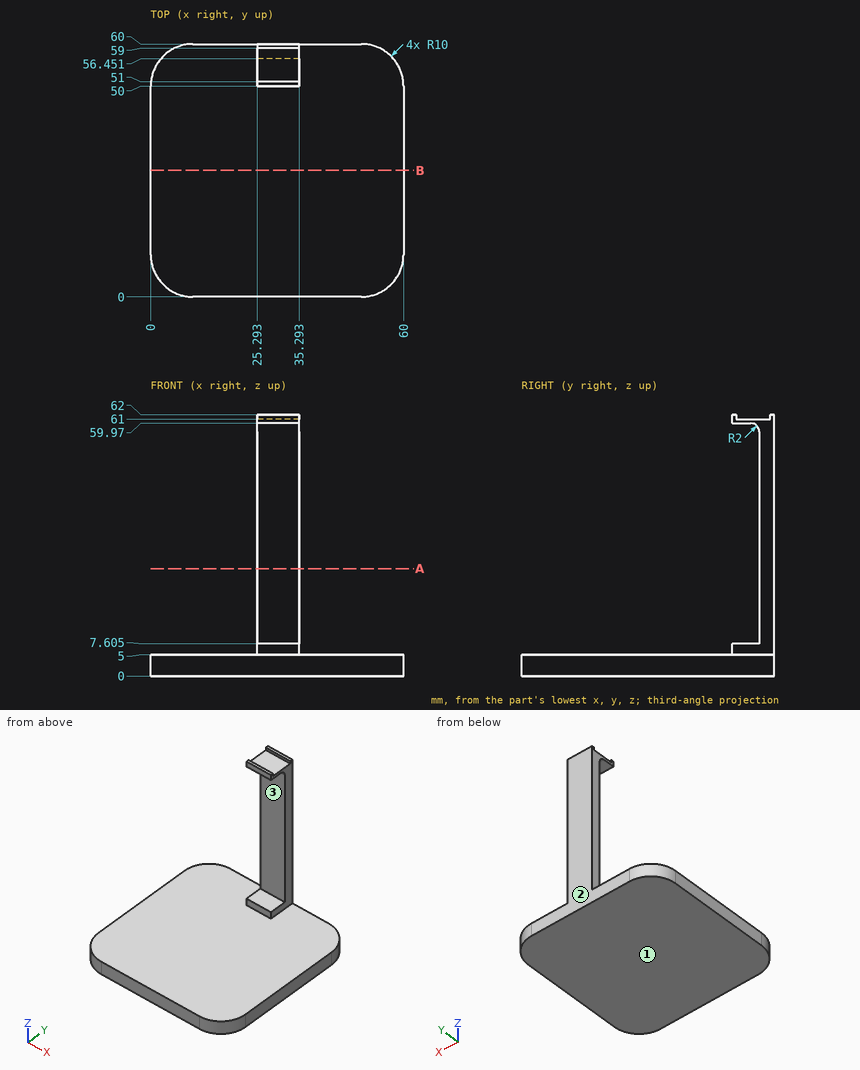
Job drawing, mm, ordinate dimensions from the low corner. One solid piece. Round coordinates to 2 decimals unless told otherwise and drop trailing zeros. Loops run counter-clockwise (first coordinate to the right, second up) from the corner with the lowest first, then second, coordinate; pieces in that order, holes last.
(1) Two-plate mould, pull along Z, no slides. Class the marked faces 1, 2 and 3: +Z half, -Z half, draft (parallel to the pull), parting line (faces both ways), or undercut.
(2) Cut at A-A (z = 25.5). Give the cut face in (x, y).
(3) Drop flat-ended pins along their axis: pin 1 (8 mm diameter, centred on x = 30.5, z = 23, fed in from -Y); pin 2 (5 mm diameter, centred on y = 53, z = 39, fed in from +X) (3 decimals); pin 3 (1.5 mm diameter, centred on x = 27, y = 53.5, fed in from +Z); pin 4 (6 mm diameter, centred on x = 47.5, y = 18.5, fed in from +Z). Give the stop position or say it passes through.
(4) Cut at B-B (y = 30). Give the cut face in (x, z), plus the area to 3 significant figures.
(5) Wall check: line 1 along Z through (x, y) = (51, 30); line 2 along Y through (x, z) = (27, 32); line 3 along Y through (x, z) = (25.5, 58.5). Give the ranges that are in metal, low to high.
Findings below:
1. face 1: -Z half
1. face 2: draft
1. face 3: undercut
2. outline: (25.29, 56.45) - (35.29, 56.45) - (35.29, 60) - (25.29, 60) - close
3. pin 1: stops at y = 56.45
3. pin 2: passes through
3. pin 3: stops at z = 61
3. pin 4: stops at z = 5
4. outline: (0, 0) - (60, 0) - (60, 5) - (0, 5) - close
4. area: 300 mm2
5. line 1: z = 0 to 5
5. line 2: y = 56.45 to 60
5. line 3: y = 56.38 to 60
